```python
from build123d import *

# Parameters (mm, degrees)
PAD002_DEPTH    = 1.95
SKETCH008_R     = 2
PAD003_DEPTH    = 1.6
SKETCH009_W     = 1.4
SKETCH009_H     = 4.2
POCKET005_DEPTH = 1.5
SKETCH010_W     = 1.3
SKETCH010_H     = 4
POCKET006_DEPTH = 0.5


with BuildPart() as part:
    # Sketch007 → Pad002 (new body)
    with BuildSketch(Plane.XZ):
        with BuildLine():
            ThreePointArc((-2.5, 2.1), (-4.6, 0), (-2.5, -2.1))
            Line((-2.5, -2.1), (2.5, -2.1))
            ThreePointArc((2.5, -2.1), (4.6, 0), (2.5, 2.1))
            Line((2.5, 2.1), (-2.5, 2.1))
        make_face()
    extrude(amount=PAD002_DEPTH)

    # Sketch008 (on Face6 of Pad002) → Pad003 (join)
    with BuildSketch(Plane.XZ.offset(1.95)):
        Circle(SKETCH008_R)
    extrude(amount=PAD003_DEPTH)

    # Sketch009 (on Face4 of Pad003) → Pocket005 (cut)
    with BuildSketch(Plane(origin=(0, 0, 0), x_dir=(1, 0, 0), z_dir=(0, 1, 0))):
        Rectangle(SKETCH009_W, SKETCH009_H)
    extrude(amount=-POCKET005_DEPTH, mode=Mode.SUBTRACT)

    # Sketch010 (on Face12 of Pocket005) → Pocket006 (cut)
    with BuildSketch(Plane.XZ.offset(3.55)):
        Rectangle(SKETCH010_W, SKETCH010_H)
    extrude(amount=-POCKET006_DEPTH, mode=Mode.SUBTRACT)


with BuildPart() as part_1:
    # Body001 placement: moved
    add(part.part.moved(Location((-4.066, -15.05, 12.2))))


solid = part_1.part
```
CAD build for the part. Positions are in the model's coordinates, mm. A direction names the side the tool comes from. Round coordinates to 2 decimals unless told otherwise and drop trailing zeros. Write each loop counter-clockwise with the first axis right and the second up, starting at its lowest first coordinate (ties: lowest second). Pieces come first, ordered by that corner, then holes.
Item 1: Band-saw the part on A-A on y = -15.75. Write the cut outline in (x, z), then the cut area to 3 significant figures.
Filled in:
outline: (-6.57, 10.1) - (-4.77, 10.1) - (-4.77, 14.3) - (-6.57, 14.3) arc R2.1 ccw to start; (-3.37, 10.1) - (-1.57, 10.1) arc R2.1 ccw to (-1.57, 14.3) - (-3.37, 14.3) - close
area: 29.0 mm2
Item 2: Band-saw the part on C-C on x = -2.5. Write the cut outline in (y, z), then the cut area to 3 significant figures.
Filled in:
outline: (-18.6, 10.96) - (-17, 10.96) - (-17, 10.1) - (-15.05, 10.1) - (-15.05, 14.3) - (-17, 14.3) - (-17, 13.44) - (-18.6, 13.44) - close
area: 12.2 mm2
Item 3: Drop flat-ended pins along their axis: pin 1 Ø1.5 at (x, z) = (-7, 11.5) entering from -Y; pin 2 Ø0.7 at (x, z) = (-4.5, 11.5) entering from +Y; pin 3 Ø0.8 at (y, z) = (-16, 11.5) entering from +X. Give the stop position or say it passes through.
Filled in:
pin 1: stops at y = -17
pin 2: stops at y = -15.05
pin 3: stops at x = 0.51
Item 4: Drill centre lines: L1, parallel to Y at x = -6, z = 13.6; L2, parallel to X at y = -17.95, z = 12.2; L3, parallel to Y at x = -3.5, z = 11. Where is each one in solid material? Low to high.
Filled in:
L1: y = -17 to -15.05
L2: x = -6.07 to -2.07
L3: y = -18.1 to -16.55
Item 5: Band-saw the part on D-D on y = -17.75. Write the cut outline in (x, z).
Filled in:
outline: circle Ø4 at (-4.07, 12.2)
Item 6: Band-saw the part on B-B on z = 12.2. Write the cut outline in (x, y), then the cut area to 3 significant figures.
Filled in:
outline: (-8.67, -17) - (-6.07, -17) - (-6.07, -18.6) - (-4.72, -18.6) - (-4.72, -18.1) - (-3.42, -18.1) - (-3.42, -18.6) - (-2.07, -18.6) - (-2.07, -17) - (0.53, -17) - (0.53, -15.05) - (-3.37, -15.05) - (-3.37, -16.55) - (-4.77, -16.55) - (-4.77, -15.05) - (-8.67, -15.05) - close
area: 21.6 mm2
Item 7: Tool access for faces 4 (the flat face through (-4, -16.55, 12)), 5 (the cylindrical face through (-8.665, -16.011, 12.246)), 6 (the flat face through (-4, -18.1, 12)): list every direction of +Z, -Z, +X, -X, +Y, -Y with a clear straight run to the whole face (end or side of a thin tool).
Filled in:
face 4: +Z, -Z, +Y
face 5: -X, +Y, -Y
face 6: +Z, -Z, -Y
Item 8: Mould opens along X. For faces 1 (the flat face through (-3.366, -16, 12)), 2 (the cylindrical face through (-2.22, -17.79, 11.43)), 3 (the flat face through (-1, -15.05, 12)) say: released by +X, released by -X, zero draft, split by the parting line, or undercut.
Filled in:
face 1: undercut
face 2: split by the parting line
face 3: zero draft
